```python
from build123d import *

# Parameters (mm, degrees)
SKETCH_W        = 64.8
SKETCH_H        = 94
PAD_DEPTH       = 55
SKETCH001_W     = 54.8
SKETCH001_H     = 84
POCKET_DEPTH    = 50
SKETCH002_R     = 2
POCKET001_DEPTH = 5
SKETCH003_W     = 10
SKETCH003_H     = 5
POCKET002_DEPTH = 5.001


with BuildPart() as part:
    # Sketch → Pad (new body)
    with BuildSketch(Plane.XZ):
        with Locations((32.4, 47)):
            Rectangle(SKETCH_W, SKETCH_H)
    extrude(amount=PAD_DEPTH)

    # Sketch001 (on Face6 of Pad) → Pocket (cut)
    with BuildSketch(Plane.XZ.offset(55)):
        with Locations((32.4, 47)):
            Rectangle(SKETCH001_W, SKETCH001_H)
    extrude(amount=-POCKET_DEPTH, mode=Mode.SUBTRACT)

    # Sketch002 (on Face5 of Pocket) → Pocket001 (cut)
    with BuildSketch(Plane.XZ.offset(55)):
        with Locations((2.5, 2.5)):
            Circle(SKETCH002_R)
        with Locations((62.3, 2.5)):
            Circle(SKETCH002_R)
        with Locations((62.3, 91.5)):
            Circle(SKETCH002_R)
        with Locations((2.5, 91.5)):
            Circle(SKETCH002_R)
    extrude(amount=-POCKET001_DEPTH, mode=Mode.SUBTRACT)

    # Sketch003 (on Face18 of Pocket001) → Pocket002 (cut, through all)
    with BuildSketch(Plane.XZ.offset(5)):
        with Locations((10, 7.5)):
            Rectangle(SKETCH003_W, SKETCH003_H)
    extrude(amount=-POCKET002_DEPTH, mode=Mode.SUBTRACT)


solid = part.part
```
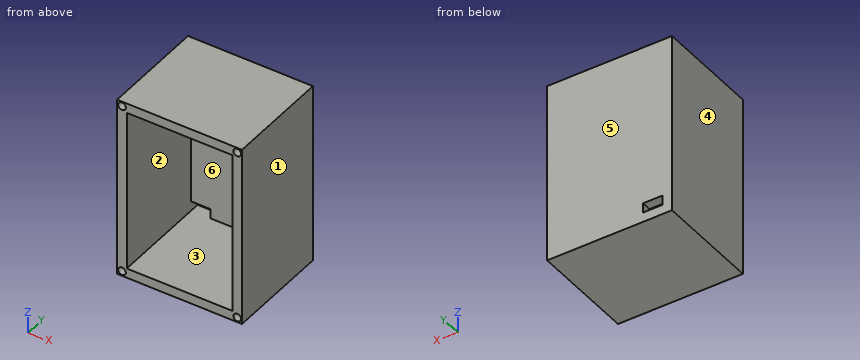
Build history of the part. All positions in model axes, mm. Face numbers are marked on the shaded views. A direction names the side the tool comes from. Round coordinates to 2 decimals unless told otherwise and drop trailing zeros. Write each loop counter-clockwise with the first axis right and the second up, starting at its lowest first coordinate (ties: lowest second). Pieces come first, ordered by that corner, then holes.
1) Band-saw the part on B-B, the plane x = 56. List the corners of the cut face in (y, z).
2) Band-saw the part on C-C, the plane z = 75.5. List the corners of the cut face in (x, y).
3) Mould opens along X. For the marked faces 3, 4, 5 and 6 say: +X half, -X half, draft (parallel to the pull), parting line (faces both ways), or undercut.
4) 3-axis set-ups, long thin cutter, end or side, ignore diameter. For the marked faces 1 and 2: which of +Z, -Z, +X, -X, +Y, -Y reach the whole face in a straight line?
5) Drill centre lines: probe 1 along Z at (x, y) = (50, -32.5); probe 2 along Z at (x, y) = (2, -51); probe 3 along X at (y, z) = (-48, 80). Where is each one in solid material? Low to high.
6) Pin check, flat tips, straight feed: pin 1 (2 mm diameter, centred on x = 63, z = 2.5, fed in from -Y); pin 2 (6 mm diameter, centred on x = 18, z = 33, fed in from -Y). Stop position of each tip, or through.
7) Band-saw the part on A-A, the plane y = -35. List the corners of the cut face in (x, z), and give its area (3 significant figures).
Ans:
1. outline: (-55, 0) - (0, 0) - (0, 94) - (-55, 94) - (-55, 89) - (-5, 89) - (-5, 5) - (-55, 5) - close
2. outline: (0, -55) - (5, -55) - (5, -5) - (59.8, -5) - (59.8, -55) - (64.8, -55) - (64.8, 0) - (0, 0) - close
3. face 3: undercut
3. face 4: -X half
3. face 5: draft
3. face 6: undercut
4. face 1: +Z, -Z, +X, +Y, -Y
4. face 2: -Y
5. probe 1: z = 0 to 5, 89 to 94
5. probe 2: z = 0 to 0.56, 4.44 to 89.56, 93.44 to 94
5. probe 3: x = 0 to 5, 59.8 to 64.8
6. pin 1: stops at y = -50
6. pin 2: stops at y = -5
7. outline: (0, 0) - (64.8, 0) - (64.8, 94) - (0, 94) - close; hole (5, 5) - (59.8, 5) - (59.8, 89) - (5, 89) - close
7. area: 1,490 mm2
